from build123d import *

# Parameters (mm, degrees)
F0_W = 100
F0_H = 100
F4_T = -4


with BuildPart() as f3:
    # F0 (on Top) → F3 section 0
    with BuildSketch(Plane.XY, mode=Mode.PRIVATE) as f3_s0:
        Rectangle(F0_W, F0_H)
    loft([f3_s0.sketch, Vertex(0, 0, 100)])

    # F4
    f4_openings = [f3.faces().sort_by_distance(p)[0] for p in [
        (0, 0, 0),
    ]]
    offset(amount=F4_T, openings=f4_openings)


solid = f3.part
Check sheet for the modelled part. Datum: model origin and axes. Units: mm. A direction names the side the tool comes from. Round coordinates to 2 decimals unless told otherwise and drop trailing zeros. Order: outer loops, then holes, each group sorted by start corner. A loop starts at its lowest first (then second) coordinate and runs counter-clockwise, first axis right, second up.
(1) Cross-section at A-A, the plane z = 41.5. Enter the section's corners in (x, y), and give its area (3 significant figures).
(2) Cross-section at B-B, the plane x = -41. Enter the section's corners in (y, z), and give its area (3 significant figures).
(3) Access from +Z, -Z, +X, -X, +Y, -Y to the whole of each face (thin tool, end or side, straight path). Record for faces 1 (the flat face through (27.504, -0.637, 36.048)), 2 (the flat face through (1, 30, 40)).
(4) Scan lines: probe 1 along Y at (x, z) = (-28, 9.5); probe 2 along Y at (x, z) = (11, 23.5); probe 3 along Z at (x, y) = (5.5, -31). Record each from-to range of solid material in increasing order.
(5) Draft check along X on faces 3 (the flat face through (-1, -30, 40)), 4 (the flat face through (-27.504, 0.637, 36.048)), 5 (the flat face through (30, -1, 40)). Enter one of: pulls with the +X half, pulls with the -X half, needs draft (parallel to the pull), parting line crosses it, or undercut.
(6) Cross-section at C-C, the plane z = 21.5. Enter the section's corners in (x, y).
(7) Cross-section at D-D, the plane y = -29.5. Enter the section's corners in (x, z).
(8) Go/stop test with flat-tipped pins: P1, Ø6, axis at x = 37, y = 30.5, coming from the +Z side; P2, Ø1.5, axis at x = -19.5, y = -22, coming from the +Z side; P3, Ø10, axis at x = 7, y = 27, coming from the -Z side. Record where each tip stops, or that it passes through.
Check sheet entries:
1. outline: (-29.25, -29.25) - (29.25, -29.25) - (29.25, 29.25) - (-29.25, 29.25) - close; hole (-24.78, -24.78) - (24.78, -24.78) - (24.78, 24.78) - (-24.78, 24.78) - close
1. area: 966 mm2
2. outline: (-50, 0) - (-45.53, 0) - (-41, 9.06) - (41, 9.06) - (45.53, 0) - (50, 0) - (41, 18) - (-41, 18) - close
2. area: 854 mm2
3. face 1: -Z
3. face 2: +Z, +X, -X, +Y
4. probe 1: y = -45.25 to -40.78, 40.78 to 45.25
4. probe 2: y = -38.25 to -33.78, 33.78 to 38.25
4. probe 3: z = 29.06 to 38
5. face 3: needs draft
5. face 4: undercut
5. face 5: pulls with the +X half
6. outline: (-39.25, -39.25) - (39.25, -39.25) - (39.25, 39.25) - (-39.25, 39.25) - close; hole (-34.78, -34.78) - (34.78, -34.78) - (34.78, 34.78) - (-34.78, 34.78) - close
7. outline: (-50, 0) - (-45.53, 0) - (-29.5, 32.06) - (29.5, 32.06) - (45.53, 0) - (50, 0) - (29.5, 41) - (-29.5, 41) - close
8. P1: stops at z = 32
8. P2: stops at z = 57.5
8. P3: stops at z = 27.06
